Input: dimensioned drawing with shaded views. Units: mm. Origin: part minimum x, y, z. Round coordinates to 2 decimals unless told otherwise and drop trailing zeros. Loops run counter-clockwise (first coordinate to the right, second up) from the corner with the lowest first, then second, coordinate; pieces in that order, holes last. Notation, with made-up numbers: M 71.25,-13.75 L 128.25,-13.75 A32 ccw 128.25,23.25 Z; hole C 19.5,86 d7. An arc over 180 degrees is marked long. Answer as a JSON object with one key per item and string values.
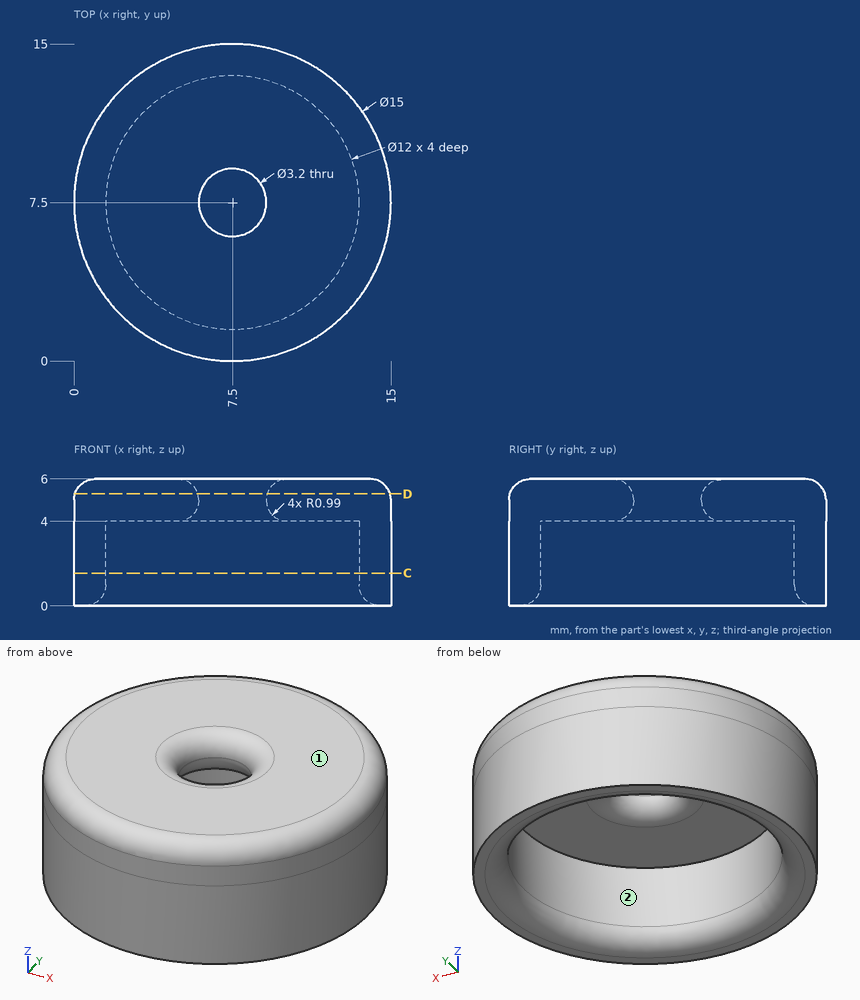
Item 1: Section D-D on z = 5.3. Return the cut outline in (x, y), then the cut area to 3 significant figures.
Answer sheet:
{"outline": "C 7.5,7.5 d14.91; hole C 7.5,7.5 d3.29", "area": "166 mm²"}
Item 2: Section C-C on z = 1.55. Return the cut outline in (x, y), then the cut area to 3 significant figures.
Answer sheet:
{"outline": "C 7.5,7.5 d15; hole C 7.5,7.5 d12", "area": "63.6 mm²"}
Item 3: Contact query for flat-ended pins moving along their axis: pin 1 Ø5 at (x, y) = (10.5, 9) entering from -Z; pin 2 Ø2 at (y, z) = (4, 1.5) entering from +X; pin 3 Ø1.5 at (y, z) = (12, 1.5) entering from -X. Output: stop coordinate, or through.
Answer sheet:
{"pin 1": "stops at z = 4", "pin 2": "stops at x = 14.57", "pin 3": "stops at x = 1"}
Item 4: Line query: probe 1 along Y at (x, z) = (7.5, 5); probe 2 along Z at (x, y) = (9, 11.5); probe 3 along Y at (x, z) = (9.5, 0.4). Output: solid intervals per line, ascending. Write a range as from..to.
Answer sheet:
{"probe 1": "y = 0..5.9, 9.1..15", "probe 2": "z = 4..6", "probe 3": "y = 0.27..1.64, 13.36..14.73"}
Item 5: Pull-direction query (Y, two-part tool) for the marked faces 1 and 2; classes: pulls with the +Y half, pulls with the -Y half, needs draft (parallel to the pull), parting line crosses it, or undercut.
Answer sheet:
{"face 1": "needs draft", "face 2": "undercut"}
